Part print with two shaded views. Sizes in mm from the minimum x, y, z corner. Coordinates: 2 decimals unless noted, no trailing zeros. Write each loop counter-clockwise with the first axis right and the second up, starting at its lowest first coordinate (ties: lowest second). Pieces come first, ordered by that corner, then holes.
Q1. Band-saw the part on A-A, the plane y = 1. Write the cut outline in (x, z), plus the area to 3 significant figures.
Q2. Band-saw the part on B-B, the plane x = 29. Write the cut outline in (y, z).
Q3. Pin check, flat tip, straight feed: P1, Ø2.5, axis at x = 103.64, z = 2.5, coming from the +Y side. Stop position of the tip, or through.
Q4. Drill centre lines: probe 1 along X at (y, z) = (0.95, 2.5); probe 2 along X at (y, z) = (0.4, 1.9); probe 3 along Z at (x, y) = (35, 0.7). Where is each one in solid material? Low to high.
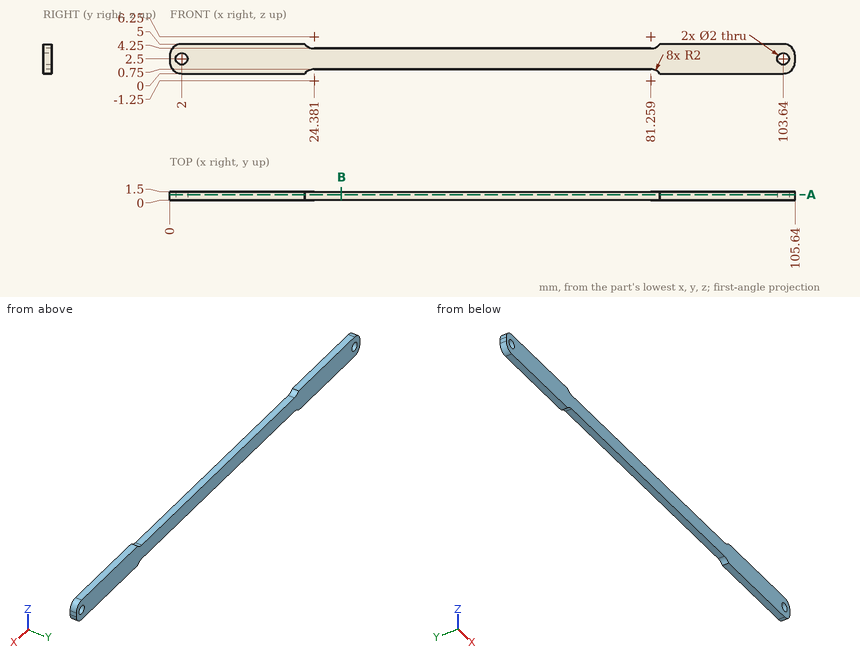
Answer sheet:
1. outline: (0, 2) arc R2 ccw to (2, 0) - (22.82, 0) arc R2 cw to (24.38, 0.75) - (81.26, 0.75) arc R2 cw to (82.82, 0) - (103.64, 0) arc R2 ccw to (105.64, 2) - (105.64, 3) arc R2 ccw to (103.64, 5) - (82.82, 5) arc R2 cw to (81.26, 4.25) - (24.38, 4.25) arc R2 cw to (22.82, 5) - (2, 5) arc R2 ccw to (0, 3) - close; hole circle Ø2 at (2, 2.5); hole circle Ø2 at (103.64, 2.5)
1. area: 430 mm2
2. outline: (0, 0.75) - (1.5, 0.75) - (1.5, 4.25) - (0, 4.25) - close
3. P1: stops at y = 1.5
4. probe 1: x = 0 to 1, 3 to 102.64, 104.64 to 105.64
4. probe 2: x = 0 to 1.2, 2.8 to 102.84, 104.44 to 105.64
4. probe 3: z = 0.75 to 4.25
